from build123d import *

# Parameters (mm, degrees)
SKETCH1_R           = 3.175
SKETCH1_W           = 5.842
SKETCH1_H           = 12.7
BOSS_EXTRUDE1_DEPTH = 5.842
FILLET3_R           = 12.7
FILLET4_R           = 1
FILLET5_R           = 1
BOSS_EXTRUDE2_DEPTH = 5.842
CUT_EXTRUDE1_DEPTH  = 282.950775489
FILLET6_R           = 6.35
BOSS_EXTRUDE3_DEPTH = 5.842


with BuildPart() as part:
    # Sketch1 → Boss-Extrude1 (new body)
    with BuildSketch(Plane.XY):
        with BuildLine():
            Line((217.770203729, 9.126532246), (220.945203729, 9.126532246))
            Line((220.945203729, 9.126532246), (220.945203729, 14.968532246))
            Line((220.945203729, 14.968532246), (233.645203729, 14.968532246))
            Line((233.645203729, 14.968532246), (233.645203729, 9.126532246))
            Line((233.645203729, 9.126532246), (236.820203729, 9.126532246))
            Line((236.820203729, 9.126532246), (248.922907622, 29.883396652))
            Line((248.922907622, 29.883396652), (248.922907622, 36.233396652))
            Line((248.922907622, 36.233396652), (248.922907622, 99.733396652))
            Line((248.922907622, 99.733396652), (248.922907622, 119.585663985))
            ThreePointArc((248.922907622, 119.585663985), (244.199339956, 129.46830165), (233.542352153, 131.99955227))
            Line((233.542352153, 131.99955227), (145.982629888, 113.092608128))
            ThreePointArc((145.982629888, 113.092608128), (141.008772871, 106.211718626), (147.322907622, 100.535663985))
            Line((147.322907622, 100.535663985), (176.730316466, 106.885663985))
            Line((176.730316466, 106.885663985), (223.522907622, 106.885663985))
            Line((223.522907622, 106.885663985), (223.522907622, 30.685663985))
            Line((223.522907622, 30.685663985), (222.929875834, 31.278695773))
            Line((222.929875834, 31.278695773), (218.798958018, 27.147777957))
            Line((218.798958018, 27.147777957), (209.818701897, 36.128034078))
            Line((209.818701897, 36.128034078), (213.949619713, 40.258951894))
            Line((213.949619713, 40.258951894), (204.969363592, 49.239208015))
            Line((204.969363592, 49.239208015), (200.838445776, 45.108290199))
            Line((200.838445776, 45.108290199), (187.961093383, 57.985642593))
            Line((187.961093383, 57.985642593), (192.092011199, 62.116560408))
            Line((192.092011199, 62.116560408), (187.601883138, 66.606688469))
            Line((187.601883138, 66.606688469), (180.072011297, 59.076816628))
            Line((180.072011297, 59.076816628), (186.339307306, 40.55742867))
            Line((186.339307306, 40.55742867), (190.829435366, 36.067300609))
            Line((190.829435366, 36.067300609), (217.770203729, 9.126532246))
        make_face()
        with Locations((236.222907622, 119.585663985)):
            Circle(SKETCH1_R, mode=Mode.SUBTRACT)
        Polygon((223.522907622, 116.989680814), (223.522907622, 113.235663985), (206.137725309, 113.235663985), align=None, mode=Mode.SUBTRACT)
        with BuildLine():
            Line((146.652768755, 109.989136056), (171.480545327, 115.350246995))
            ThreePointArc((171.480545327, 115.350246995), (175.254156266, 112.916913791), (172.820823062, 109.143302852))
            Line((172.820823062, 109.143302852), (147.99304649, 103.782191913))
            ThreePointArc((147.99304649, 103.782191913), (144.219435551, 106.215525117), (146.652768755, 109.989136056))
        make_face(mode=Mode.SUBTRACT)
        with BuildLine():
            Line((183.894433613, 118.030802464), (208.722210185, 123.391913403))
            ThreePointArc((208.722210185, 123.391913403), (212.495821124, 120.958580199), (210.062487919, 117.18496926))
            Line((210.062487919, 117.18496926), (185.234711348, 111.823858321))
            ThreePointArc((185.234711348, 111.823858321), (181.461100409, 114.257191525), (183.894433613, 118.030802464))
        make_face(mode=Mode.SUBTRACT)
        with Locations((236.222907622, 38.956098115)):
            Rectangle(SKETCH1_W, SKETCH1_H, mode=Mode.SUBTRACT)
        with Locations((236.222907622, 64.356098115)):
            Rectangle(SKETCH1_W, SKETCH1_H, mode=Mode.SUBTRACT)
        with Locations((236.222907622, 89.756098115)):
            Rectangle(SKETCH1_W, SKETCH1_H, mode=Mode.SUBTRACT)
    extrude(amount=BOSS_EXTRUDE1_DEPTH)

    # Fillet3
    # the kernel refuses this fillet: 12.7 mm, written as the material it adds along each edge
    with BuildSketch(Plane(origin=(223.522907622, 106.885663985, 0), x_dir=(0, -1, 0), z_dir=(0, 0, 1))) as fillet3_piece_1:
        with BuildLine():
            CenterArc((FILLET3_R, -FILLET3_R), FILLET3_R, 90, 90)
            Line((0, -FILLET3_R), (0, 0))
            Line((0, 0), (FILLET3_R, 0))
        make_face()
    extrude(amount=5.842)
    with BuildSketch(Plane(origin=(176.730316466, 106.885663985, 0), x_dir=(1, 0, 0), z_dir=(0, 0, 1))) as fillet3_piece_2:
        with BuildLine():
            CenterArc((FILLET3_R * 0.106735979666, -FILLET3_R), FILLET3_R, 90, 12.184909582)
            Line((-FILLET3_R * 0.104331380131, -FILLET3_R * 0.0225284814234), (0, 0))
            Line((0, 0), (FILLET3_R * 0.106735979666, 0))
        make_face()
    extrude(amount=5.842)
    # the kernel refuses this fillet: 12.7 mm, written as the material it takes off along each edge
    with BuildSketch(Plane(origin=(248.922907622, 29.883396652, -8.580237273), x_dir=(-0.50370125175659, -0.8638779132370756, 0), z_dir=(0, 0, 1))) as fillet3_2_piece_1:
        with BuildLine():
            CenterArc((FILLET3_R * 0.270243693634, -FILLET3_R), FILLET3_R, 90, 30.245176455)
            Line((-FILLET3_R * 0.233457558122, -FILLET3_R * 0.136122086763), (0, 0))
            Line((0, 0), (FILLET3_R * 0.270243693634, 0))
        make_face()
    extrude(amount=23.002474546, mode=Mode.SUBTRACT)
    with BuildSketch(Plane(origin=(217.770203729, 9.126532246, -12.412377003), x_dir=(1, 0, 0), z_dir=(0, 0, 1))) as fillet3_2_piece_2:
        with BuildLine():
            CenterArc((5.469505741, 12.491006501), FILLET3_R, 225, 34.591227114)
            Line((-3.51075038, 3.51075038), (0, 0))
            Line((0, 0), (3.175, 0))
        make_face()
    extrude(amount=30.666754006, mode=Mode.SUBTRACT)

    # Fillet4
    fillet4_edges = [part.edges().sort_by_distance(p)[0] for p in [
        (223.522907622, 116.989680814, 2.921),
        (206.137725309, 113.235663985, 2.921),
        (223.522907622, 113.235663985, 2.921),
    ]]
    fillet(fillet4_edges, radius=FILLET4_R)

    # Fillet5
    # the kernel refuses this fillet: 1 mm, written as the material it adds along each edge
    with BuildSketch(Plane(origin=(223.522907622, 30.685663985, 0), x_dir=(0, 1, 0), z_dir=(0, 0, 1))) as fillet5_piece_1:
        with BuildLine():
            CenterArc((1.50647411, 1), FILLET5_R, 204.01452435, 65.98547565)
            Line((0.593031788, 0.593031788), (0.574762942, 0.584892424))
            ThreePointArc((0.574762942, 0.584892424), (0.282373759, 0.31065803), (-0.014142136, 0.014142136))
            Line((-0.014142136, 0.014142136), (0, -0.02))
            Line((0, -0.02), (1.50647411, -0.02))
            Line((1.50647411, -0.02), (1.50647411, 0))
        make_face()
    extrude(amount=5.842)

    # Sketch4 → Boss-Extrude2 (add)
    with BuildSketch(Plane.XY.offset(5.842)):
        Polygon((192.092011199, 62.116560408), (222.590849502, 31.617722105), (222.929875834, 31.278695773), (218.798958018, 27.147777957), (187.961093383, 57.985642593), align=None)
    extrude(amount=-BOSS_EXTRUDE2_DEPTH)

    # Sketch5 → Cut-Extrude1 (cut, through all)
    with BuildSketch(Plane.XY.offset(5.842)):
        Polygon((191.912406076, 52.956699165), (187.781488261, 48.825781349), (196.761744382, 39.845525228), (200.892662197, 43.976443044), align=None)
        Polygon((209.872918318, 34.996186923), (205.742000503, 30.865269107), (214.722256624, 21.885012986), (218.85317444, 26.015930802), align=None)
    extrude(amount=-CUT_EXTRUDE1_DEPTH, mode=Mode.SUBTRACT)

    # Fillet6
    fillet6_edges = [part.edges().sort_by_distance(p)[0] for p in [
        (186.339307306, 40.55742867, 2.921),
        (180.072011297, 59.076816628, 2.921),
        (187.601883138, 66.606688469, 2.921),
    ]]
    fillet(fillet6_edges, radius=FILLET6_R)

    # Sketch6 → Boss-Extrude3 (add)
    with BuildSketch(Plane.XY.offset(5.842)):
        Polygon((168.804107439, 99.197497251), (156.390219153, 96.516941781), (155.157163637, 102.227330393), (167.571051923, 104.907885862), align=None)
    extrude(amount=-BOSS_EXTRUDE3_DEPTH)


solid = part.part
Model file for the job. Use its own axes, mm. A direction names the side the tool comes from. Coordinates: 2 decimals unless noted, no trailing zeros. Write each loop counter-clockwise with the first axis right and the second up, starting at its lowest first coordinate (ties: lowest second). Pieces come first, ordered by that corner, then holes. Notation, with made-up numbers: (-32, 7) -> (-28, 7) arc R34 cw to (-28, 37) -> close; hole circle Ø3 at (-27.5, 25). An arc over 180 degrees is marked (long way). One line per item, written item: value. Start each with the question number.
1) Slice it at A-A on y = 92.5. Write the cut outline in (x, z), then the cut area to 3 significant figures.
2) Pull direction X, two halves, no side cores. Call faces 1 (the face through (220.945, 12, 3)), 2 (the face through (207.836, 32.96, 2.962)), 3 (the face through (248.47, 29.96, 2.88)), 4 (the face through (227, 76, 5.842)): +X half, -X half, draft (parallel to the pull), parting line (faces both ways), or undercut.
3) Which spindle directions (+Z, -Z, +X, -X, +Y, -Y) get a long thin tool onto all of the face, cutting with end or side? Do faces 5 (the face through (196.135, 120.674, 2.88)), 6 (the face through (181.18, 58.87, 2.96)), 7 (the face through (233.645, 12, 3)). Say none if no direction does.
4) Probe probe 1 along Y at (x, z) = (203, 2.5); probe 2 along X at (y, z) = (59, 3.1); probe 3 along Y at (x, z) = (191.5, 4.5). List the from-to ranges inside material, lowest first.
5) Slice it at D-D on z = 4.55. Count the separate pieces of the cut face and the enclosed holes in it, then the cut area to 3 significant figures.
6) Slice it at C-C on x = 162. Write the cut outline in (y, z).
7) Slice it at B-B on y = 60. Write the cut outline in (x, z).
8) Flat gauge pins, fed straight in: pin 1 Ø3 at (y, z) = (90, 4) entering from -X; pin 2 Ø1.8 at (x, z) = (200, 2.5) entering from -Y; pin 3 Ø1.8 at (y, z) = (11.5, 4) entering from +X. Where does each tip first touch, or does it go through?
Answers follow:
1. outline: (223.52, 0) -> (233.3, 0) -> (233.3, 5.84) -> (223.52, 5.84) -> close; (239.14, 0) -> (248.92, 0) -> (248.92, 5.84) -> (239.14, 5.84) -> close
1. area: 114 mm2
2. face 1: undercut
2. face 2: undercut
2. face 3: +X half
2. face 4: draft
3. face 5: +Z, -Z
3. face 6: +Z, -Z, -X
3. face 7: +Z, -Z, -Y
4. probe 1: 23.9 to 51.21, 106.89 to 115.66, 122.16 to 125.4
4. probe 2: 181.21 to 195.21, 223.52 to 233.3, 239.14 to 248.92
4. probe 3: 35.4 to 45.11, 52.54 to 62.64, 106.89 to 113.18, 119.67 to 122.92
5. separate pieces: 1
5. enclosed holes: 9
5. area: 4,510 mm2
6. outline: (97.73, 0) -> (106.81, 0) -> (106.81, 5.84) -> (97.73, 5.84) -> close; (113.3, 0) -> (116.55, 0) -> (116.55, 5.84) -> (113.3, 5.84) -> close
7. outline: (181.57, 0) -> (194.21, 0) -> (194.21, 5.84) -> (181.57, 5.84) -> close; (223.52, 0) -> (233.3, 0) -> (233.3, 5.84) -> (223.52, 5.84) -> close; (239.14, 0) -> (248.92, 0) -> (248.92, 5.84) -> (239.14, 5.84) -> close
8. pin 1: x = 223.52
8. pin 2: y = 26
8. pin 3: x = 238.73
